For this review, take the finished solid that the model builds, in its own axes (mm). A direction names the side the tool comes from. Give positions to 0.01 mm unless a question says otherwise; leave off trailing zeros. Write each loop counter-clockwise with the first axis right and the second up, starting at its lowest first coordinate (ties: lowest second). Pieces come first, ordered by that corner, then holes.
Q1. We need section D-D (x = -3.25). Write out the cut boundary in (y, z), then the cut area to 3 significant figures.
Q2. For line 1 (Y direction, x = -3.25, z = 3.5); line 2 (Y direction, x = 3, z = 6); line 3 (X direction, y = 21.75, z = 13.5), list the stretches that pass through material, from the lowest coordinate up.
Q3. Machinability: for faces 1 (the flat face through (-25, 1, 5)), 2 (the flat face through (0, 1, 10)), 3 (the flat face through (-5, -1, 0)), which of the approach directions +Z, -Z, +X, -X, +Y, -Y give a long, thin tool a straight path to every point of the face, cutting with its end or side? Answer none if there is none.
Q4. We need section C-C (z = -70). Write out the cut boundary in (x, y).
Q5. Insertion check: P1, Ø24, axis at x = -45, y = 16, coming from the -Z side; P2, Ø5.5, axis at x = -3.25, y = 21.75, coming from the +Z side; P3, Ø3, axis at y = 20.5, z = 4.5, coming from the +X side; P4, Ø3, axis at x = -36.75, y = 28.25, coming from the -Z side. Each pin has a flat end and moves straight along its axis. Give the tip position at first contact, or say it passes through.
Q6. We need section B-B (y = -28.25). Write out the cut boundary in (x, z).
Q7. We need section A-A (x = 20). Write out the cut boundary in (y, z), then the cut area to 3 significant figures.
Q8. Mouldability with a two-part tool opening along Y and no side actions: class faces 4 (the cylindrical face through (3.2, -26.5, 4.9)), 5 (the cylindrical face through (19.474, -55.14, -68.331)), 6 (the flat face through (-6, -65, -31)) as released by +Y, released by -Y, zero draft, split by the parting line, or undercut.
Autodesk Inventor part; units mm, degrees
ref_plane "YZ Plane" through (0, 0, 0) normal (1, 0, 0) x (0, 1, 0)
ref_plane "XZ Plane" through (0, 0, 0) normal (0, 1, 0) x (-1, 0, 0)
ref_plane "XY Plane" through (0, 0, 0) normal (0, 0, 1) x (1, 0, 0)
sketch "Boceto1" plane through (0, 0, 0) normal (0, 0, 1) x (1, 0, 0)
  line L0 (-15, 45) -> (15, 45)
  line L1 (15, 45) -> (15, -45)
  line L2 (15, -45) -> (-15, -45)
  line L3 (-15, -45) -> (-15, 45)
  line L4 (-15, 45) -> (15, -45) construction
  line L5 (15, 45) -> (-15, -45) construction
  point P0 (0, 0)
  dimension "d0" = 30
  dimension "d1" = 90
extrude "Extrusión1" add sketch "Boceto1" along normal blind 10
sketch "Boceto2" plane through (0, 0, 10) normal (0, 0, 1) x (1, 0, 0)
  line L0 (15, 45) -> (15, -45)
  line L1 (5, 30) -> (5, 20)
  line L2 (-5, 30) -> (5, 30)
  line L3 (5, 20) -> (-5, 30) construction
  line L4 (5, 20) -> (-5, 20)
  line L5 (-5, 20) -> (5, 30) construction
  line L6 (-5, 20) -> (-5, 30)
  line L7 (24, 0) -> (9, 0)
  line L8 (-15, -45) -> (15, -45)
  line L9 (5, 25) -> (5.4102, 25)
  circle A0 centre (-3.25, 21.75) radius 1.75
  circle A1 centre (3.25, 28.25) radius 1.75
  line L10 (5, -20) -> (-5, -20)
  circle A2 centre (-3.25, -21.75) radius 1.75
  line L11 (5, -25) -> (5.4102, -25)
  line L12 (5, -30) -> (5, -20)
  line L13 (-5, -30) -> (5, -30)
  line L14 (5, -20) -> (-5, -30) construction
  line L15 (-5, -20) -> (5, -30) construction
  line L16 (-5, -20) -> (-5, -30)
  circle A3 centre (3.25, -28.25) radius 1.75
  line L17 (-15, -45) -> (-15, 45)
  line L18 (15, -45) -> (15, 45)
  line L19 (-15, -45) -> (15, -45)
  line L20 (-15, 45) -> (15, 45)
  line L21 (-3.25, 28.25) -> (3.25, 21.75)
  line L22 (-3.25, 21.75) -> (3.25, 28.25)
  point P0 (0, 0)
  point P1 (-113, 215)
  point P2 (-5, 25)
  point P3 (-3.25, -21.75)
  point P4 (3.25, -28.25)
  point P5 (-143, 115)
  point P6 (-3.25, -21.75)
  point P7 (-5, -25)
  point P8 (3.25, -28.25)
  point P9 (0, 25)
  point P10 (0, -25)
  dimension "d4" = 1.75
  dimension "d5" = 1.75
  dimension "d6" = 1.75
  dimension "d7" = 1.75
  dimension "d8" = 10
  dimension "d9" = 10
  dimension "d10" = 10
  dimension "d11" = 15
  dimension "d12" = 0
  dimension "d13" = 30
  dimension "d14" = 0
  dimension "d15" = 90
  dimension "d16" = 15
hole "Agujero1" at (3.25, 28.25, 10) at (-3.25, 21.75, 10) at (-3.25, -21.75, 10) at (3.25, -28.25, 10) direction (0, 0, -1) diameter 3.5 end through all
sketch "Boceto3" plane through (-15, -45, 0) normal (-1, 0, 0) x (0, 0, 1)
  line L0 (0, 0) -> (0, 90)
  line L1 (0, 90) -> (20, 90)
  line L2 (20, 90) -> (20, 0)
  line L3 (20, 0) -> (0, 0)
  line L4 (0, 0) -> (0, 90)
  point P0 (0, 45)
  dimension "d24" = 20
  dimension "d25" = 90
extrude "Extrusión2" add sketch "Boceto3" along normal blind 10
sketch "Boceto4" plane through (-25, -45, 0) normal (-1, 0, 0) x (0, 0, 1)
  line L0 (20, 90) -> (10, 90)
  line L1 (10, 0) -> (10, 90)
  line L2 (20, 90) -> (10, 90)
  line L3 (10, 90) -> (10, 0)
  line L4 (10, 0) -> (20, 0)
  line L5 (20, 0) -> (20, 90)
  point P0 (0, 45)
extrude "Extrusión3" add sketch "Boceto4" along normal blind 30
sketch "Boceto5" plane through (-15, -45, 20) normal (0, 0, 1) x (1, 0, 0)
  line L0 (-40, 0) -> (-70, 90)
  line L1 (-70, 90) -> (-40, 0)
  line L2 (-20, 75) -> (-20, 65)
  line L3 (-30, 75) -> (-20, 75)
  line L4 (-20, 65) -> (-30, 75) construction
  line L5 (-20, 65) -> (-30, 65)
  line L6 (-30, 65) -> (-20, 75) construction
  circle A0 centre (-28.25, 66.75) radius 1.75
  line L7 (-30, 65) -> (-30, 75)
  circle A1 centre (-21.75, 73.25) radius 1.75
  line L8 (-40, -20) -> (-40, 90)
  line L9 (-55, 45) -> (-143, 45)
  line L10 (-20, 25) -> (-30, 25)
  circle A2 centre (-28.25, 23.25) radius 1.75
  line L11 (-20, 15) -> (-20, 25)
  line L12 (-20, 25) -> (-30, 15) construction
  line L13 (-30, 25) -> (-20, 15) construction
  line L14 (-30, 25) -> (-30, 15)
  line L15 (-30, 15) -> (-20, 15)
  circle A3 centre (-21.75, 16.75) radius 1.75
  line L16 (-70, 0) -> (-40, 0)
  line L17 (0, 0) -> (-40, 0)
  line L18 (-40, 90) -> (-70, 90)
  line L19 (-40, 0) -> (-40, 90)
  point P0 (15, 45)
  point P1 (-30, 70)
  point P2 (-20, 70)
  point P3 (-20, 20)
  point P4 (-30, 20)
  point P5 (-55, 0)
  point P6 (-55, 90)
  dimension "d30" = 3.5
  dimension "d31" = 1.75
  dimension "d32" = 1.75
  dimension "d33" = 1.75
  dimension "d34" = 1.75
  dimension "d35" = 10
  dimension "d36" = 10
  dimension "d38" = 10
  dimension "d39" = -41.1096
  dimension "d40" = 15
  dimension "d41" = 0
  dimension "d42" = 15
  dimension "d43" = 90
  dimension "d45" = 0
hole "Agujero2" at (-36.75, 28.25, 20) at (-43.25, 21.75, 20) at (-43.25, -21.75, 20) at (-36.75, -28.25, 20) direction (0, 0, -1) diameter 3.5 end through all
sketch "Boceto6" plane through (-15, -45, 20) normal (0, 0, 1) x (1, 0, 0)
  line L0 (-10, 0) -> (-40, 0)
  line L1 (-40, 0) -> (60, 0)
  line L2 (60, 0) -> (60, -20)
  line L3 (60, -20) -> (-40, -20)
  line L4 (-40, -20) -> (-40, 0)
  point P0 (15, 45)
  dimension "d53" = 20
extrude "Extrusión4" add sketch "Boceto6" against normal blind 100
mirror "Simetría1" about plane through (-5, -55, -80) normal (0, 0, -1) of "Extrusión1", "Agujero1", "Extrusión2", "Agujero2", "Extrusión3", "Extrusión4"
ref_plane "Plano de trabajo2" through (45, -65, -80) normal (0, 0, -1) x (-1, 0, 0)
sketch "Boceto7" plane through (-15, -45, 20) normal (0, 1, 0) x (1, 0, 0)
  line L0 (30, 115) -> (30, 85)
  circle A0 centre (35, 90) radius 1.75
  line L1 (30, 85) -> (40, 85)
  line L2 (35, 110) -> (35, 90)
  circle A1 centre (35, 110) radius 1.75
  line L3 (40, 115) -> (30, 85) construction
  line L4 (40, 115) -> (30, 115)
  line L5 (30, 115) -> (40, 85) construction
  line L6 (40, 85) -> (40, 115)
  line L7 (60, 0) -> (60, 200)
  line L8 (-40, 0) -> (60, 0)
  line L9 (10, 0) -> (10, 134.4524)
  line L10 (-10, 115) -> (-10, 85)
  circle A2 centre (-15, 110) radius 1.75
  line L11 (-20, 115) -> (-10, 115)
  circle A3 centre (-15, 90) radius 1.75
  line L12 (-10, 85) -> (-20, 85)
  line L13 (-20, 115) -> (-10, 85) construction
  line L14 (-10, 115) -> (-20, 85) construction
  line L15 (-20, 85) -> (-20, 115)
  line L16 (-15, 110) -> (-15, 90)
  point P0 (15, 20)
  point P1 (189.1833, 40)
  point P2 (35, 115)
  point P3 (-85.8367, 100)
  point P4 (235.02, 100)
  point P5 (-15, 115)
  dimension "d56" = 5
  dimension "d57" = 5
  dimension "d58" = 3.5
  dimension "d59" = 5
  dimension "d60" = 5
  dimension "d61" = 10
  dimension "d62" = 30
  dimension "d64" = 20
hole "Agujero3" at (-30, -45, -90) at (-30, -45, -70) at (20, -45, -90) at (20, -45, -70) direction (0, -1, 0) diameter 3.5 end through all
split "Dividir1" plane through (45, -65, -80) removes the side toward (0, 0, -1)
properties part number "container_mid_2"
Computed:
1. outline: (-65, -80) - (-45, -80) - (-45, 0) - (-23.5, 0) - (-23.5, 10) - (-45, 10) - (-45, 20) - (-65, 20) - close; (-20, 0) - (20, 0) - (20, 10) - (-20, 10) - close; (23.5, 0) - (45, 0) - (45, 10) - (23.5, 10) - close
1. area: 2,830 mm2
2. line 1: y = -65 to -23.5, -20 to 20, 23.5 to 45
2. line 2: y = -65 to -29.98, -26.52 to 26.52, 29.98 to 45
2. line 3: x = -55 to -45, -41.5 to -15
3. face 1: -Z, -X, +Y
3. face 2: +Z, +X, +Y
3. face 3: -Z, +X, -X, +Y
4. outline: (-55, -65) - (-31.75, -65) - (-31.75, -45) - (-55, -45) - close; (-28.25, -65) - (18.25, -65) - (18.25, -45) - (-28.25, -45) - close; (21.75, -65) - (45, -65) - (45, -45) - (21.75, -45) - close
5. P1: stops at z = 10
5. P2: stops at z = 10
5. P3: stops at x = 15
5. P4: passes through
6. outline: (-55, 10) - (-38.5, 10) - (-38.5, 20) - (-55, 20) - close; (-35, 10) - (-25, 10) - (-25, 0) - (1.5, 0) - (1.5, 10) - (-15, 10) - (-15, 20) - (-35, 20) - close; (5, 0) - (15, 0) - (15, 10) - (5, 10) - close
7. outline: (-65, -80) - (-45, -80) - (-45, -71.75) - (-65, -71.75) - close; (-65, -68.25) - (-45, -68.25) - (-45, 20) - (-65, 20) - close
7. area: 1,930 mm2
8. face 4: undercut
8. face 5: zero draft
8. face 6: released by -Y
